```python
from build123d import *

# Parameters (mm, degrees)
EXTRUDE_1_DEPTH     = 41
CUT_EXTRUDE_1_REACH = 59.313
SKETCH_2_R          = 3.3
CUT_EXTRUDE_2_REACH = 58.815
SKETCH_3_R          = 6.4
SKETCH_4_R          = 2.47
EXTRUDE_2_DEPTH     = 5
CHAMFER_1_SIZE      = 0.5
FILLET_1_R          = 0.5
EXTRUDE_3_DEPTH     = 10
CUT_EXTRUDE_3_DEPTH = 4
CUT_EXTRUDE_4_REACH = 59.297
SKETCH_7_R          = 1.65
FILLET_2_R          = 3


with BuildPart() as part:
    # 草图1 → 凸台-拉伸1 (new body)
    with BuildSketch(Plane.XY):
        Polygon((0, 0), (5, 0), (5, 39), (-4.099065175, 39), align=None)
    extrude(amount=EXTRUDE_1_DEPTH)

    # 切除-拉伸1: up to this plane
    cut_extrude_1_end = Plane(origin=(0, 0, 41), z_dir=(0.9945218953682742, 0.10452846326764682, 0))
    # 草图2 → 切除-拉伸1 (cut, up to the surface)
    with BuildSketch(Plane(origin=(5, 0, 0), x_dir=(0, 0, -1), z_dir=(1, 0, 0)), mode=Mode.PRIVATE) as cut_extrude_1_sk1:
        with Locations(Location((-29.5, 22, 0), (0, 0, 90))):
            Circle(SKETCH_2_R)
    cut_extrude_1_tool1 = split(extrude(cut_extrude_1_sk1.sketch, amount=-CUT_EXTRUDE_1_REACH, mode=Mode.PRIVATE), bisect_by=cut_extrude_1_end, keep=Keep.BOTH, mode=Mode.PRIVATE)
    add(cut_extrude_1_tool1.solids().sort_by_distance((5, 22, 29.5))[0], mode=Mode.SUBTRACT)

    # 切除-拉伸2: up to this plane
    cut_extrude_2_end = Plane(origin=(0, 0, 41), z_dir=(0.9945218953682742, 0.10452846326764682, 0))
    # 草图3 → 切除-拉伸2 (cut, up to the surface)
    with BuildSketch(Plane.ZY.offset(-1), mode=Mode.PRIVATE) as cut_extrude_2_sk1:
        with Locations(Location((29.5, 22, 0), (0, 0, 270))):
            Circle(SKETCH_3_R)
    cut_extrude_2_tool1 = split(extrude(cut_extrude_2_sk1.sketch, amount=CUT_EXTRUDE_2_REACH, mode=Mode.PRIVATE), bisect_by=cut_extrude_2_end, keep=Keep.BOTH, mode=Mode.PRIVATE)
    add(cut_extrude_2_tool1.solids().sort_by_distance((1, 22, 29.5))[0], mode=Mode.SUBTRACT)

    # 草图4 → 凸台-拉伸2 (add)
    with BuildSketch(Plane(origin=(5, 0, 0), x_dir=(0, 0, -1), z_dir=(1, 0, 0))):
        with Locations(Location((-29.5, 36, 0), (0, 0, 270))):
            Circle(SKETCH_4_R)
    extrude(amount=EXTRUDE_2_DEPTH)

    # 倒角1
    chamfer_1_edges = [part.edges().sort_by_distance(p)[0] for p in [
        (10, 38.47, 29.5),
    ]]
    chamfer(chamfer_1_edges, length=CHAMFER_1_SIZE)

    # 圆角1
    fillet_1_edges = [part.edges().sort_by_distance(p)[0] for p in [
        (5, 38.47, 29.5),
    ]]
    fillet(fillet_1_edges, radius=FILLET_1_R)

    # 草图5 → 凸台-拉伸3 (add)
    with BuildSketch(Plane(origin=(0, 0, 0), x_dir=(-1, 0, 0), z_dir=(0, 0, -1))):
        Polygon((-5, 32), (3.363335529, 32), (0.735729647, 7), (-5, 7), align=None)
    extrude(amount=EXTRUDE_3_DEPTH)

    # 草图6 → 切除-拉伸3 (cut)
    with BuildSketch(Plane(origin=(5, 0, 0), x_dir=(0, 0, -1), z_dir=(1, 0, 0))):
        Polygon((8.175426481, 27), (6.58771324, 29.75), (3.41228676, 29.75), (1.824573519, 27), (3.41228676, 24.25), (6.58771324, 24.25), align=None)
        Polygon((8.175426481, 12), (6.58771324, 14.75), (3.41228676, 14.75), (1.824573519, 12), (3.41228676, 9.25), (6.58771324, 9.25), align=None)
    extrude(amount=-CUT_EXTRUDE_3_DEPTH, mode=Mode.SUBTRACT)

    # 切除-拉伸4: up to this plane
    cut_extrude_4_end = Plane(origin=(0, 0, 41), z_dir=(0.9945218953682742, 0.10452846326764682, 0))
    # 草图7 → 切除-拉伸4 (cut, up to the surface)
    with BuildSketch(Plane(origin=(1, 0, 0), x_dir=(0, 0, -1), z_dir=(1, 0, 0)), mode=Mode.PRIVATE) as cut_extrude_4_sk1:
        with Locations((5, 27)):
            Circle(SKETCH_7_R)
    cut_extrude_4_tool1 = split(extrude(cut_extrude_4_sk1.sketch, amount=-CUT_EXTRUDE_4_REACH, mode=Mode.PRIVATE), bisect_by=cut_extrude_4_end, keep=Keep.BOTH, mode=Mode.PRIVATE)
    add(cut_extrude_4_tool1.solids().sort_by_distance((1, 27, -5))[0], mode=Mode.SUBTRACT)
    # 草图7 → 切除-拉伸4 (cut, up to the surface)
    with BuildSketch(Plane(origin=(1, 0, 0), x_dir=(0, 0, -1), z_dir=(1, 0, 0)), mode=Mode.PRIVATE) as cut_extrude_4_sk2:
        with Locations((5, 12)):
            Circle(SKETCH_7_R)
    cut_extrude_4_tool2 = split(extrude(cut_extrude_4_sk2.sketch, amount=-CUT_EXTRUDE_4_REACH, mode=Mode.PRIVATE), bisect_by=cut_extrude_4_end, keep=Keep.BOTH, mode=Mode.PRIVATE)
    add(cut_extrude_4_tool2.solids().sort_by_distance((1, 12, -5))[0], mode=Mode.SUBTRACT)

    # 圆角2
    fillet_2_edges = [part.edges().sort_by_distance(p)[0] for p in [
        (0.450467412, 39, 41),
        (2.132135177, 7, 0),
        (0.818332236, 32, 0),
        (2.132135177, 7, -10),
        (0.818332236, 32, -10),
        (0.450467412, 39, 0),
        (2.5, 0, 0),
        (2.5, 0, 41),
    ]]
    fillet(fillet_2_edges, radius=FILLET_2_R)


solid = part.part
```
Geometry check sheet. Reference: the model listing, model coordinates, mm. A direction names the side the tool comes from. Coordinates: 2 decimals unless noted, no trailing zeros. Write each loop counter-clockwise with the first axis right and the second up, starting at its lowest first coordinate (ties: lowest second). Pieces come first, ordered by that corner, then holes. Notation, with made-up numbers: M 19.25,1 L 46.25,1 A30 ccw 46.25,28 Z; hole C -7.5,-15 d11. An arc over 180 degrees is marked long. One line per item, written item: value. Start each with the question number.
(1) Sectioned sample at D-D, the plane z = 24.5. Enter the section's corners in (x, y) (3 decimals).
(2) Depth check by flat-ended pin: pin 1 (3 mm diameter, centred on y = 34, z = 1, fed in from -X); pin 2 (1.2 mm diameter, centred on x = 2.5, z = -4.5, fed in from -Y); pin 3 (10 mm diameter, centred on y = 23.5, z = 32.5, fed in from -X); pin 4 (2 mm diameter, centred on x = 7.5, z = 35.5, fed in from -Y). Enter the tip coordinate at first touch or a pass-through.
(3) Tool access check on faces 4 (the face through (2.3, 3.5, 0)), 5 (the face through (0.5, 35.5, 0)), 6 (the face through (3.03, 25.64, -2.61)). Record the directions out of +Z, -Z, +X, -X, +Y, -Y that give a thin tool (end or side, any length) a straight path to the whole face; none if there is none.
(4) Sectioned sample at A-A, the plane x = 4.25. State how many separate pieces and enclosed holes the cut face has, and give its area (3 significant figures).
(5) Scan lines: line 1 along Y through (x, z) = (2.25, -6.5); line 2 along Z through (x, y) = (-0.05, 12); line 3 along Y through (x, z) = (0.35, -5). Record each from-to range of solid material in increasing order. Write a range as [from, to].
(6) Sectioned sample at C-C, the plane y = 22. Enter the section's corners in (x, z), and give its area (3 significant figures).
(7) Release check for a two-part mould opening along Z. For faces 1 (the face through (2.38, 0.86, 0.9)), 2 (the face through (2, 20, 41)), 3 (the face through (3.03, 28.36, -7.39)) record: released by +Z, released by -Z, zero draft, split by the parting line, or undercut.
(8) Sectioned sample at B-B, the plane z = -5. Enter the section's corners in (x, y), and give its area (3 significant figures).
Filled sheet:
1. outline: M -4.099,39 L -2.732,25.995 L 1,25.995 L 1,18.005 L -1.892,18.005 L 0,0 L 5,0 L 5,39 Z
2. pin 1: x = -3.73
2. pin 2: y = 7
2. pin 3: x = -3
2. pin 4: through
3. face 4: -Z, +X, -X, -Y
3. face 5: -Z, +X, -X, +Y
3. face 6: +X
4. separate pieces: 1
4. enclosed holes: 3
4. area: 1,750 mm²
5. line 1: [7, 9.25], [14.75, 24.25], [29.75, 32]
5. line 2: [-10, -6.65], [-3.35, 41]
5. line 3: [7, 10.35], [13.65, 25.35], [28.65, 32]
6. outline: M -2.31,-10 L 5,-10 L 5,26.2 L 1,26.2 L 1,23.1 L -2.31,23.1 Z; M -2.31,35.9 L 1,35.9 L 1,32.8 L 5,32.8 L 5,41 L -2.31,41 Z
6. area: 304 mm²
7. face 1: released by -Z
7. face 2: released by +Z
7. face 3: undercut
8. outline: M -3.36,32 L -3.01,28.65 L 1,28.65 L 1,29.75 L 5,29.75 L 5,32 Z; M -2.66,25.35 L -1.43,13.65 L 1,13.65 L 1,14.75 L 5,14.75 L 5,24.25 L 1,24.25 L 1,25.35 Z; M -1.09,10.35 L -0.74,7 L 5,7 L 5,9.25 L 1,9.25 L 1,10.35 Z
8. area: 112 mm²
